Build history of the part. All positions in model axes, mm. Face numbers are marked on the shaded views. A direction names the side the tool comes from. Round coordinates to 2 decimals unless told otherwise and drop trailing zeros. Loops run counter-clockwise (first coordinate to the right, second up) from the corner with the lowest first, then second, coordinate; pieces in that order, holes last. Notation, with made-up numbers: M 10,70 L 68,70 A10 cw 68,82 Z; hole C 5,64.5 d1. An arc over 180 degrees is marked long. Write each question's results on one line, items separated by ' | '. Start each with the question number.
Autodesk Inventor part; units mm, degrees
ref_plane "YZ Plane" through (0, 0, 0) normal (1, 0, 0) x (0, 1, 0)
ref_plane "XZ Plane" through (0, 0, 0) normal (0, 1, 0) x (-1, 0, 0)
ref_plane "XY Plane" through (0, 0, 0) normal (0, 0, 1) x (1, 0, 0)
sketch "Sketch1" plane through (0, 0, 0) normal (0, 1, 0) x (-1, 0, 0)
  circle A0 centre (0, 0) radius 6.45
  circle A1 centre (0, 0) radius 5.657
  circle A2 centre (0, 0) radius 2.85
  circle A3 centre (0, 0) radius 1.5
  line L0 (0, 0) -> (-36, 0)
  circle A4 centre (-36, 0) radius 3.5
  line L1 (0, 6.45) -> (-36, 3.5)
  line L2 (0, -6.45) -> (-36, -3.5)
  dimension "d0" = 12.9
  dimension "d1" = 11.314
  dimension "d2" = 5.7
  dimension "d3" = 3
  dimension "d4" = 36
  dimension "d5" = 7
extrude "Extrusion1" add sketch "Sketch1" along normal blind 2 contours A0 L2 L1 | A0 L0 A4 L1 | L2 A4 L0 A0 | A4
sketch "Sketch2" plane through (0, 2, 0) normal (0, 1, 0) x (1, 0, 0)
  line L0 (8.4358, -5.7587) -> (8.4358, 5.7587)
  line L1 (8.4358, -5.7587) -> (0, -6.45)
  line L2 (0, -6.45) -> (36, -3.5)
  line L3 (8.4358, 5.7587) -> (0, 6.45)
  line L4 (36, 3.5) -> (0, 6.45)
  arc A0 (0, 6.45) -> (0, -6.45) centre (0, 0) ccw
  arc A1 (0, 6.45) -> (0, -6.45) centre (0, 0) ccw
  circle A2 centre (0, 0) radius 5.657
extrude "Extrusion2" add sketch "Sketch2" along normal blind 1.5
fillet "Fillet1" radius 10 1 edges at (8.4358, 3.5, 0)
sketch "Sketch4" plane through (0, 2, 0) normal (0, 1, 0) x (1, 0, 0)
  circle A0 centre (0, 0) radius 2.9
  circle A1 centre (0, 0) radius 1.5
  dimension "d11" = 5.8
  dimension "d12" = 3
sketch "Sketch5" plane through (0, 2, 0) normal (0, 1, 0) x (1, 0, 0)
  circle A0 centre (0, 0) radius 5.657
extrude "Extrusion3" add sketch "Sketch5" along normal blind 0.5 and the other way blind 3
sketch "Sketch6" plane through (0, 2.5, 0) normal (0, 1, 0) x (1, 0, 0)
  circle A0 centre (0, 0) radius 2.9
  dimension "d17" = 5.8
extrude "Extrusion4" cut sketch "Sketch6" against normal blind 0.5
hole "Hole1" at (0, 2, 0) direction (0, -1, 0) diameter 3 end through all
sketch "Sketch7" plane through (0, -1, 0) normal (0, -1, 0) x (1, 0, 0)
  circle A0 centre (0, 0) radius 2.9
  dimension "d27" = 5.8
hole "Hole2" at (0, -1, 0) direction (0, 1, 0) diameter 5.8 depth 2 tip angle 118
sketch "Sketch9" plane through (0, 2, 0) normal (0, 1, 0) x (1, 0, 0)
  line L0 (8.4358, 5.7587) -> (8.4358, -5.7587)
  arc A0 (36, -3.5) -> (36, 3.5) centre (36, 0) ccw
  circle A1 centre (23.9679, 0) radius 1
  circle A2 centre (34.612, 0) radius 1
  line L1 (0, -6.45) -> (36, -3.5)
  circle A3 centre (29.29, 0) radius 1
  circle A4 centre (13.3238, 0) radius 1
  circle A5 centre (18.6459, 0) radius 1
  point P0 (0, 0)
hole "Hole4" at (13.3238, 2, 0) at (18.6459, 2, 0) at (23.9679, 2, 0) at (29.29, 2, 0) at (34.612, 2, 0) direction (0, -1, 0) diameter 2 end through all
properties part number "servo_arm_2"
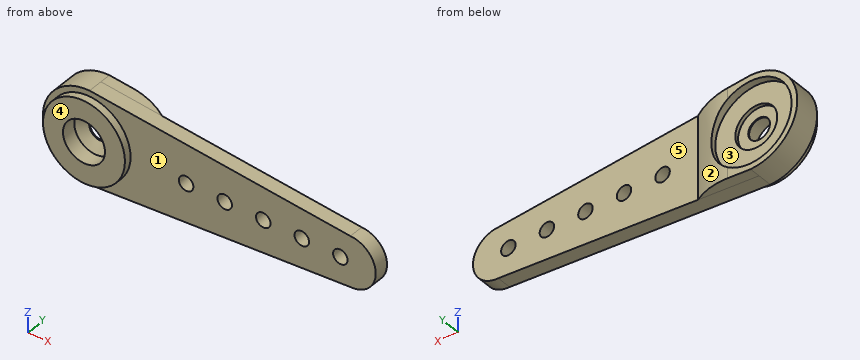
Item 1: Drop flat-ended pins along their axis: pin 1 (2.5 mm diameter, centred on x = 23.97, z = 0, fed in from -Y); pin 2 (2.5 mm diameter, centred on x = 0, z = 0, fed in from +Y); pin 3 (1.7 mm diameter, centred on x = -0.5, z = -0.5, fed in from +Y); pin 4 (3.5 mm diameter, centred on x = -2, z = -0.5, fed in from +Y). Give the stop position or say it passes through.
Item 2: Tool access for the marked faces 4 and 5: list every direction of +Z, -Z, +X, -X, +Y, -Y with a clear straight run to the whole face (end or side of a thin tool).
Item 3: Saw through at A-A, the plane x = 29.29. Give the cut face in (y, z).
Item 4: Mould opens along X. For the marked faces 1, 2 and 3 say: released by +X, released by -X, zero draft, split by the parting line, or undercut.
Item 5: Drill centre lines: line 1 along Z through (x, y) = (0, 3.35); line 2 along Z through (x, y) = (0, 0.05); line 3 along X through (y, z) = (-0.1, 0). Where is each one in solid material? Low to high. Write a range as [from, to].
Item 6: Saw through at C-C, the plane x = 7.5. Give the cut face in (y, z).
Item 7: Saw through at B-B, the plane z = 0. State how many separate pieces and enclosed holes the cut face has, then the cut area to 3 significant figures.
Working result:
1) pin 1: stops at y = 0 | pin 2: passes through | pin 3: stops at y = 2 | pin 4: stops at y = 2.5
2) face 4: +Z, -Z, +X, -X, -Y | face 5: +Z, -Z, +X, +Y
3) outline: M 0,-4.05 L 2,-4.05 L 2,-1 L 0,-1 Z; M 0,1 L 2,1 L 2,4.05 L 0,4.05 Z
4) face 1: zero draft | face 2: released by +X | face 3: undercut
5) line 1: z = [-6.45, -5.66], [5.66, 6.45] | line 2: z = [-6.45, -2.9], [2.9, 6.45] | line 3: x = [-5.66, -2.9], [2.9, 5.66]
6) outline: M 0,-5.84 L 2.51,-5.84 L 2.51,5.84 L 0,5.84 Z
7) separate pieces: 7 | enclosed holes: 0 | area: 73.3 mm²
